Part print with two shaded views. Sizes in mm from the minimum x, y, z corner. A direction names the side the tool comes from. Round coordinates to 2 decimals unless told otherwise and drop trailing zeros. Order: outer loops, then holes, each group sorted by start corner. A loop starts at its lowest first (then second) coordinate and runs counter-clockwise, first axis right, second up. Notation, with made-up numbers: (36.5, -39.75) -> (75.5, -39.75) arc R28 ccw to (75.5, -8.75) -> close; hole circle Ø10 at (10, 34.5). An arc over 180 degrees is marked (long way). Use a Markdown table: item, result. Add a question column.
Item 1: Probe L1, parallel to Y at x = 18, z = 19.5; L2, parallel to Y at x = 33, z = 14.5; L3, parallel to Y at x = 14, z = 9. List the from-to ranges inside material, lowest first.
Item 2: Slice it at C-C, the plane y = 180.5. Give the cut face in (x, z).
Item 3: 3-axis set-ups, long thin cutter, end or side, ignore diameter. For the marked faces 1, 2 and 3: which of +Z, -Z, +X, -X, +Y, -Y reach the whole face in a straight line?
Item 4: Slice it at D-D, the plane z = 13. Give the cut face in (x, y).
Item 5: Pin check, flat tips, straight feed: pin 1 (3 mm diameter, centred on x = 31, z = 24, fed in from -Y); pin 2 (3 mm diameter, centred on y = 43.5, z = 31.5, fed in from +X); pin 3 (8 mm diameter, centred on y = 183.5, z = 17.5, fed in from -X); pin 4 (9 mm diameter, centred on y = 6.5, z = 16.5, fed in from +X). Stop position of each tip, or through.
Item 6: Slice it at A-A, the plane z = 23. Give the cut face in (x, y), plus the area to 3 significant figures.
Item 7: Slice it at B-B, the plane x = 20.5. Give the cut face in (y, z) (3 decimals).
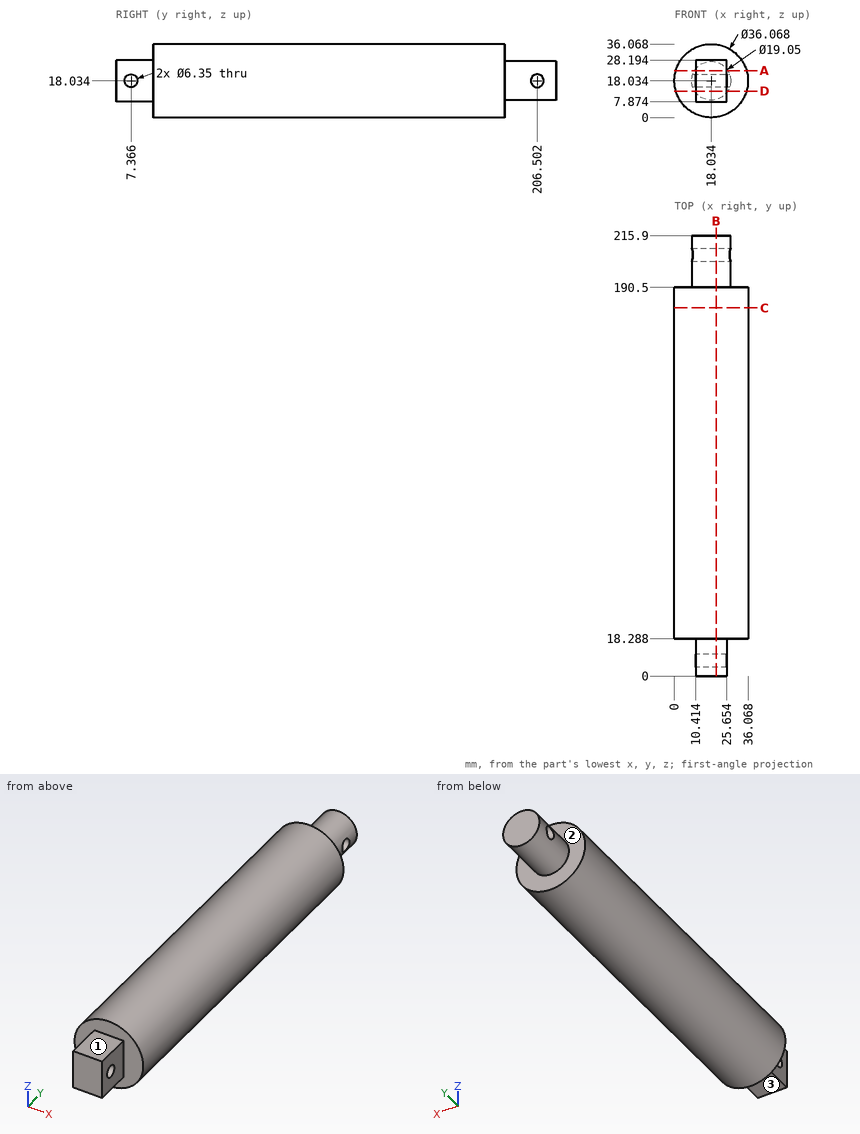
Check sheet entries:
| question | item | result |
|---|---|---|
| 1 | L1 | 0 to 4.55, 10.18 to 203.69, 209.32 to 215.9 |
| 1 | L2 | 18.29 to 190.5 |
| 1 | L3 | 0 to 190.5 |
| 2 | outline | circle Ø36.07 at (18.03, 18.03) |
| 3 | face 1 | +Z, +X, -X, -Y |
| 3 | face 2 | +Y |
| 3 | face 3 | -Z, +X, -X, -Y |
| 4 | outline | (0.72, 18.29) -> (10.41, 18.29) -> (10.41, 0) -> (25.65, 0) -> (25.65, 18.29) -> (35.35, 18.29) -> (35.35, 190.5) -> (26.12, 190.5) -> (26.12, 215.9) -> (9.95, 215.9) -> (9.95, 190.5) -> (0.72, 190.5) -> close |
| 5 | pin 1 | y = 18.29 |
| 5 | pin 2 | x = 31.53 |
| 5 | pin 3 | x = 0 |
| 5 | pin 4 | x = 25.65 |
| 6 | outline | (0.7, 18.29) -> (10.41, 18.29) -> (10.41, 0) -> (25.65, 0) -> (25.65, 18.29) -> (35.37, 18.29) -> (35.37, 190.5) -> (26.16, 190.5) -> (26.16, 215.9) -> (9.91, 215.9) -> (9.91, 190.5) -> (0.7, 190.5) -> close |
| 6 | area | 6,660 mm2 |
| 7 | outline | (0, 7.874) -> (18.288, 7.874) -> (18.288, 0.169) -> (190.5, 0.169) -> (190.5, 8.834) -> (215.9, 8.834) -> (215.9, 27.234) -> (190.5, 27.234) -> (190.5, 35.899) -> (18.288, 35.899) -> (18.288, 28.194) -> (0, 28.194) -> close; hole circle Ø6.35 at (7.366, 18.034); hole circle Ø6.35 at (206.502, 18.034) |
